The model under review builds one solid part; all positions refer to its coordinate system, in mm. Give positions to 0.01 mm unless a question says otherwise; leave off trailing zeros. Order: outer loops, then holes, each group sorted by start corner. A loop starts at its lowest first (then second) coordinate and runs counter-clockwise, first axis right, second up. Notation, with made-up numbers: (-25.75, -11) -> (21.25, -11) arc R25 ccw to (21.25, 28) -> close; hole circle Ø9 at (12, -15). An arc over 180 degrees is marked (long way). Use one line per item in the form item = value.
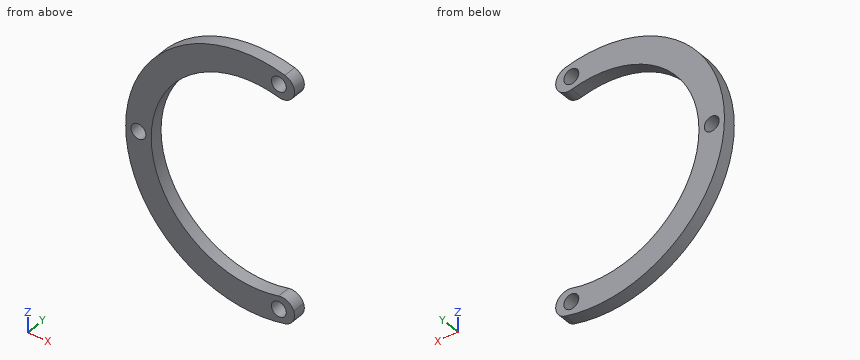
Autodesk Inventor part; units mm, degrees
ref_plane "YZ Plane" through (0, 0, 0) normal (1, 0, 0) x (0, 1, 0)
ref_plane "XZ Plane" through (0, 0, 0) normal (0, 1, 0) x (-1, 0, 0)
ref_plane "XY Plane" through (0, 0, 0) normal (0, 0, 1) x (1, 0, 0)
sketch "Sketch1" plane through (0, 0, 0) normal (0, 1, 0) x (-1, 0, 0)
  arc A0 (-10.5785, -28.0731) -> (-10.5785, 28.0731) centre (0, 0) ccw
  arc A1 (-23.5162, 13.2661) -> (-10.5785, 24.8414) centre (0, 0) ccw construction
  arc A2 (-10.5785, -21.5429) -> (-10.5785, 21.5429) centre (0, 0) ccw
  circle A3 centre (27, 0) radius 1.75
  circle A4 centre (16.8342, 21.1095) radius 1.75
  circle A5 centre (-6.0081, 26.3231) radius 1.75
  circle A6 centre (-24.3262, 11.7149) radius 1.75
  circle A7 centre (-24.3262, -11.7149) radius 1.75
  circle A8 centre (-6.0081, -26.3231) radius 1.75
  circle A9 centre (16.8342, -21.1095) radius 1.75
  line L0 (-10.5785, 28.0731) -> (-8.5262, 22.4344)
  line L1 (-10.5785, 28.0731) -> (-4.578, 28.0731) construction
  line L2 (-10.5785, -28.0731) -> (-8.5262, -22.4344)
  dimension "d2" = 60
  dimension "d3" = 54
  dimension "d4" = 48
  dimension "d5" = 3.5
  dimension "d6" = 360
  dimension "d7" = 70
extrude "Extrusion1" add sketch "Sketch1" along normal blind 3 contours L2 A2 L0 A0 | A4 | A9
fillet "Fillet1" radius 3 4 edges at (10.5785, 1.5, 28.0731) (8.5262, 1.5, 22.4344) (8.5262, 1.5, -22.4344) (10.5785, 1.5, -28.0731)
properties part number "Reverse Lever Ring" material "Copper"
1. Add section D-D on z = -8. Give the boundary of the cut face in (x, y), then the cut area to 3 significant figures.
Values:
outline = (-28.91, 0) -> (-22.63, 0) -> (-22.63, 3) -> (-28.91, 3) -> close
area = 18.9 mm^2
2. For L1, parallel to Z at x = 0, y = 0.8; L2, parallel to Z at x = -16.5, y = 0.2; L3, parallel to X at y = 2.25, z = 21.5, list the stretches that pass through material, from the lowest coordinate up.
Values:
L1 = -30 to -24, 24 to 30
L2 = -25.06 to -17.43, 17.43 to 25.06
L3 = -20.92 to -10.67
3. Add section C-C on y = 1.7. Count the separate pieces of the cut face and the enclosed holes in it, then the cut area to 3 significant figures.
Values:
separate_pieces = 1
enclosed_holes = 3
area = 589 mm^2
4. For pin 1 Ø1 at (x, y) = (-22, 1) entering from -Z; pin 2 Ø1 at (x, y) = (1.5, 2) entering from -Z, all flat-tipped, find the tip position at first contact; note any pin that passes through.
Values:
pin_1 = -20.92
pin_2 = -29.98
5. Add section B-B on z = 0. Give the boundary of the cut face in (x, y).
Values:
outline = (-30, 0) -> (-28.75, 0) -> (-28.75, 3) -> (-30, 3) -> close; (-25.25, 0) -> (-24, 0) -> (-24, 3) -> (-25.25, 3) -> close
6. Add section A-A on x = 0. Give the boundary of the cut face in (y, z), then the cut area to 3 significant figures.
Values:
outline = (0, -30) -> (3, -30) -> (3, -24) -> (0, -24) -> close; (0, 24) -> (3, 24) -> (3, 30) -> (0, 30) -> close
area = 36.0 mm^2
